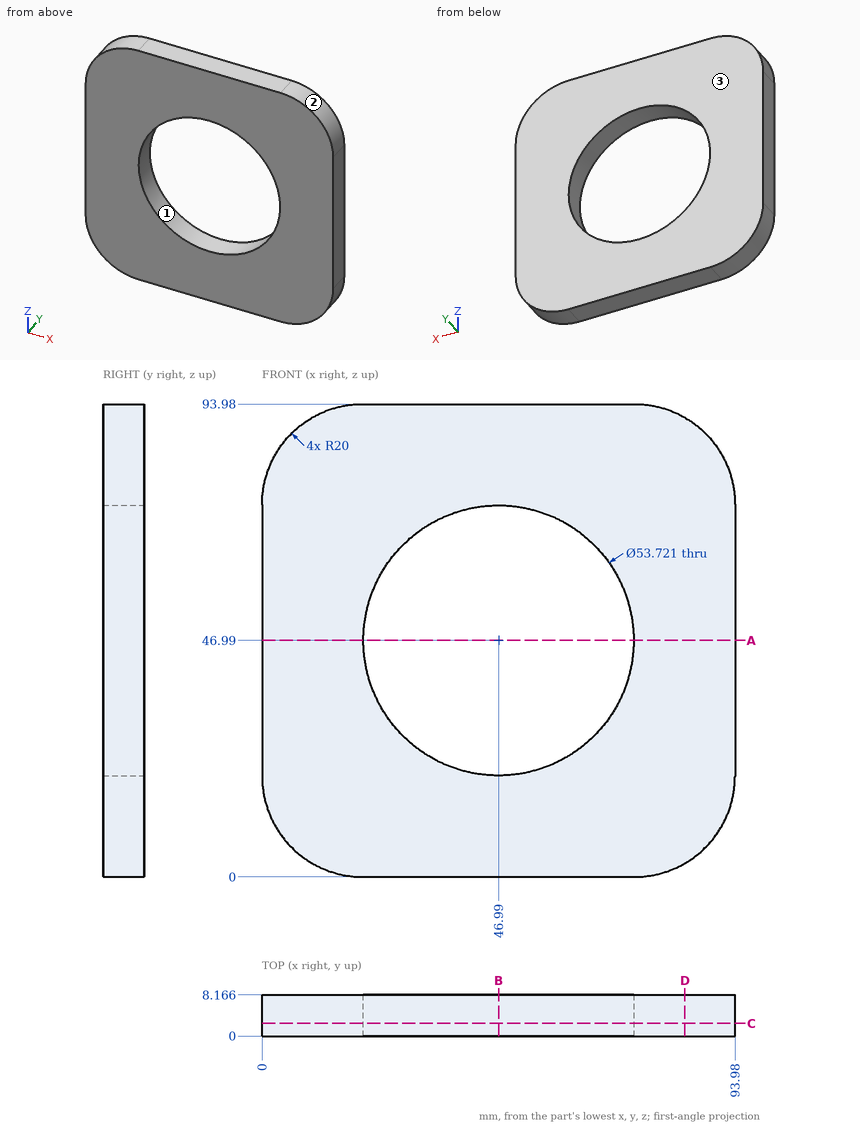
Study the drawing (mm; zero at the part's minimum x, y, z) and answer. Coordinates: 2 decimals unless noted, no trailing zeros. Loops run counter-clockwise (first coordinate to the right, second up) from the corner with the lowest first, then second, coordinate; pieces in that order, holes last. Notation, with made-up numbers: (-19.5, 45) -> (-10.5, 45) arc R21 ccw to (-10.5, 75) -> close; hole circle Ø6 at (-29.75, 70). An arc over 180 degrees is marked (long way). Write each question's results on one line, items separated by ' | '. Start each with the question number.
1) Find section B-B on x = 46.99. Determine the outline of the cut face in (y, z), then the cut area to 3 significant figures.
2) The mould has two halves that part along Z. Classify the marked faces 1, 2 and 3: pulls with the +Z half, pulls with the -Z half, needs draft (parallel to the pull), parting line crosses it, or undercut.
3) Find section A-A on z = 46.99. Determine the outline of the cut face in (x, y), then the cut area to 3 significant figures.
4) Find section D-D on x = 84. Determine the outline of the cut face in (y, z), then the cut area to 4 significant figures.
5) Consider line 1 along X through (y, z) = (1, 48); line 2 along Z through (x, y) = (46.99, 6.25); line 3 along Z through (x, y) = (65, 7). Determine where each line is inside the solid, lowest interval first.
6) Find section C-C on y = 2.5. Determine the outline of the cut face in (x, z).
Response values:
1) outline: (0, 0) -> (8.17, 0) -> (8.17, 20.13) -> (0, 20.13) -> close; (0, 73.85) -> (8.17, 73.85) -> (8.17, 93.98) -> (0, 93.98) -> close | area: 329 mm^2
2) face 1: undercut | face 2: pulls with the +Z half | face 3: needs draft
3) outline: (0, 0) -> (20.13, 0) -> (20.13, 8.17) -> (0, 8.17) -> close; (73.85, 0) -> (93.98, 0) -> (93.98, 8.17) -> (73.85, 8.17) -> close | area: 329 mm^2
4) outline: (0, 2.69) -> (8.17, 2.69) -> (8.17, 91.29) -> (0, 91.29) -> close | area: 723.5 mm^2
5) line 1: x = 0 to 20.15, 73.83 to 93.98 | line 2: z = 0 to 20.13, 73.85 to 93.98 | line 3: z = 0 to 27.06, 66.92 to 93.98
6) outline: (0, 20) arc R20 ccw to (20, 0) -> (73.98, 0) arc R20 ccw to (93.98, 20) -> (93.98, 73.98) arc R20 ccw to (73.98, 93.98) -> (20, 93.98) arc R20 ccw to (0, 73.98) -> close; hole circle Ø53.72 at (46.99, 46.99)
